Can you work these out from the model? Positions are in its coordinate system, mm. Round coordinates to 2 decimals unless told otherwise and drop trailing zeros. Order: outer loops, then holes, each group sorted by start corner. A loop starts at its lowest first (then second) coordinate and runs counter-clockwise, first axis right, second up. Notation, with made-up numbers: M 82,-18.75 L 118,-18.75 A15 cw 118,-5.75 Z; hole C -24.75,-25.75 d1. An arc over 180 degrees is marked long. One line per question, with ' | ' between items.
Autodesk Inventor part; units mm, degrees
ref_plane "YZ Plane" through (0, 0, 0) normal (1, 0, 0) x (0, 1, 0)
ref_plane "XZ Plane" through (0, 0, 0) normal (0, 1, 0) x (-1, 0, 0)
ref_plane "XY Plane" through (0, 0, 0) normal (0, 0, 1) x (1, 0, 0)
sketch "Эскиз1" plane through (0, 0, 0) normal (0, 0, 1) x (1, 0, 0)
  line L0 (74.0863, 5.032) -> (74.0863, 52.032)
  line L1 (81.155, -20.903) -> (-58.845, -20.903)
  line L2 (-58.845, -20.903) -> (-58.845, -64.903)
  line L3 (-58.845, -64.903) -> (81.155, -64.903)
  line L4 (81.155, -64.903) -> (81.155, -20.903)
  point P0 (0, 0)
  dimension "d0" = 44
  dimension "d1" = 140
extrude "Выдавливание1" add sketch "Эскиз1" along normal blind 22
fillet "Сопряжение1" radius 10 2 edges at (81.155, -42.903, 22) (81.155, -42.903, 0)
properties part number "akum12v"
(1) Please list where these lines run through material, in increasing order: probe 1 along X at (y, z) = (-43, 20.5) (3 decimals); probe 2 along X at (y, z) = (-53, 20) (3 decimals). Write a range as [from, to].
Final values:
probe 1: [-58.845, 76.423] | probe 2: [-58.845, 77.155]
(2) Will these pins go through, and if not, where does the flat tip stop? pin 1 Ø3 at (y, z) = (-48, 6) entering from +X; pin 2 Ø3 at (x, y) = (-15, -45.5) entering from -Z.
Final values:
pin 1: x = 80.84 | pin 2: z = 0
(3) If we section it at A-A on z = 3.5: Please give me the cut outline in (x, y) (3 decimals), plus the area to 3 significant figures.
Final values:
outline: M -58.845,-64.903 L 78.754,-64.903 L 78.754,-20.903 L -58.845,-20.903 Z | area: 6,050 mm^2
